from build123d import *

# Parameters (mm, degrees)
SKETCH_1_W           = 44
SKETCH_1_H           = 81
EXTRUDE_1_DEPTH      = 25
SHELL_1_T            = -2
FILLET_1_R           = 2
SKETCH_2_R           = 0.8
SKETCH_2_R_2         = 0.9
CUT_EXTRUDE_1_DEPTH  = 24
SKETCH_3_R           = 1.25
CUT_EXTRUDE_2_DEPTH  = 24
SKETCH_4_R           = 6
EXTRUDE_2_DEPTH      = 2
CUT_EXTRUDE_START    = -13.2
SKETCH_6_R           = 1.25
CUT_EXTRUDE_4_DEPTH  = 13.2
SKETCH_7_W           = 15.5
SKETCH_7_H           = 17.5
CUT_EXTRUDE_5_DEPTH  = 13.2
SKETCH_9_W           = 18.8
SKETCH_9_H           = 6.5
SKETCH_9_R           = 0.9
EXTRUDE_3_DEPTH      = 8
SKETCH_11_W          = 11
SKETCH_11_H          = 6.5
CUT_EXTRUDE_6_DEPTH  = 4
SKETCH_12_W          = 10
SKETCH_12_H          = 3.5
CUT_EXTRUDE_7_DEPTH  = 4
FILLET_2_R           = 2
EXTRUDE_START        = -1
SKETCH_14_R          = 1.25
EXTRUDE_4_DEPTH      = 1
SKETCH_15_R          = 2
CUT_EXTRUDE_8_DEPTH  = 1
SKETCH_17_R          = 2
EXTRUDE_5_DEPTH      = 3
SKETCH_18_R          = 0.85
CUT_EXTRUDE_10_DEPTH = 3
FILLET_4_R           = 1


with BuildPart() as part:
    # 草图1 → 凸台-拉伸1 (new body)
    with BuildSketch(Plane(origin=(0, 0, 0), x_dir=(1, 0, 0), z_dir=(0, 1, 0))):
        with Locations((0, -2.5)):
            Rectangle(SKETCH_1_W, SKETCH_1_H)
    extrude(amount=EXTRUDE_1_DEPTH)

    # 抽壳1
    shell_1_openings = [part.faces().sort_by_distance(p)[0] for p in [
        (0, 25, 2.5),
    ]]
    offset(amount=SHELL_1_T, openings=shell_1_openings, kind=Kind.INTERSECTION)

    # 圆角1
    fillet_1_edges = [part.edges().sort_by_distance(p)[0] for p in [
        (0, 0, -38),
        (22, 0, 2.5),
        (0, 0, 43),
        (-22, 0, 2.5),
        (-22, 12.5, -38),
        (22, 12.5, -38),
        (22, 12.5, 43),
        (-22, 12.5, 43),
    ]]
    fillet(fillet_1_edges, radius=FILLET_1_R)

    # 草图2 → 切除-拉伸1 (cut)
    with BuildSketch(Plane(origin=(0, 2, 0), x_dir=(1, 0, 0), z_dir=(0, 1, 0))):
        with Locations(Location((4.8, 16.9, 0), (0, 0, 270))):
            Circle(SKETCH_2_R)
        with Locations(Location((16.1, -9.5, 0), (0, 0, 270))):
            Circle(SKETCH_2_R_2)
    extrude(amount=-CUT_EXTRUDE_1_DEPTH, mode=Mode.SUBTRACT)

    # 草图3 → 切除-拉伸2 (cut)
    with BuildSketch(Plane(origin=(0, 2, 0), x_dir=(1, 0, 0), z_dir=(0, 1, 0))):
        with Locations(Location((-9.5, -3, 0), (0, 0, 270))):
            Circle(SKETCH_3_R)
    extrude(amount=-CUT_EXTRUDE_2_DEPTH, mode=Mode.SUBTRACT)

    # 草图4 → 凸台-拉伸2 (add)
    with BuildSketch(Plane(origin=(0, 2, 0), x_dir=(1, 0, 0), z_dir=(0, 1, 0))):
        with Locations(Location((-9.5, -3, 0), (0, 0, 270))):
            Circle(SKETCH_4_R)
    extrude(amount=EXTRUDE_2_DEPTH)

    # 草图6 → 切除-拉伸4 (cut)
    with BuildSketch(Plane.XZ.offset(CUT_EXTRUDE_START)):
        with Locations(Location((-9.5, 3, 0), (0, 0, 90))):
            Circle(SKETCH_6_R)
    extrude(amount=CUT_EXTRUDE_4_DEPTH, mode=Mode.SUBTRACT)

    # 草图7 → 切除-拉伸5 (cut)
    with BuildSketch(Plane(origin=(0, 0, -38), x_dir=(-1, 0, 0), z_dir=(0, 0, -1))):
        with Locations((-10.25, 12.5)):
            Rectangle(SKETCH_7_W, SKETCH_7_H)
    extrude(amount=-CUT_EXTRUDE_5_DEPTH, mode=Mode.SUBTRACT)

    # 草图9 → 凸台-拉伸3 (add)
    with BuildSketch(Plane(origin=(0, 2, 0), x_dir=(1, 0, 0), z_dir=(0, 1, 0))):
        with Locations((10.6, -37.75)):
            Rectangle(SKETCH_9_W, SKETCH_9_H)
        with Locations(Location((18.1, -37.9, 0), (0, 0, 270))):
            Circle(SKETCH_9_R, mode=Mode.SUBTRACT)
        with Locations(Location((3.1, -37.9, 0), (0, 0, 270))):
            Circle(SKETCH_9_R, mode=Mode.SUBTRACT)
    extrude(amount=EXTRUDE_3_DEPTH)

    # 草图11 → 切除-拉伸6 (cut)
    with BuildSketch(Plane(origin=(0, 10, 0), x_dir=(1, 0, 0), z_dir=(0, 1, 0))):
        with Locations((10.6, -37.75)):
            Rectangle(SKETCH_11_W, SKETCH_11_H)
    extrude(amount=-CUT_EXTRUDE_6_DEPTH, mode=Mode.SUBTRACT)

    # 草图12 → 切除-拉伸7 (cut)
    with BuildSketch(Plane.XY.offset(43)):
        with Locations((10.6, 10)):
            Rectangle(SKETCH_12_W, SKETCH_12_H)
    extrude(amount=-CUT_EXTRUDE_7_DEPTH, mode=Mode.SUBTRACT)

    # 圆角2
    fillet_2_edges = [part.edges().sort_by_distance(p)[0] for p in [
        (10.6, 2, 34.5),
        (1.2, 2, 37.75),
        (1.2, 6, 34.5),
    ]]
    fillet(fillet_2_edges, radius=FILLET_2_R)

    # 草图14 → 凸台-拉伸4 (add)
    with BuildSketch(Plane.XZ.offset(EXTRUDE_START)):
        with Locations(Location((-9.5, 3, 0), (0, 0, 90))):
            Circle(SKETCH_14_R)
    extrude(amount=EXTRUDE_4_DEPTH)

    # 草图15 → 切除-拉伸8 (cut)
    with BuildSketch(Plane.XZ):
        with Locations(Location((16.1, 9.5, 0), (0, 0, 270))):
            Circle(SKETCH_15_R)
        with Locations(Location((4.8, -16.9, 0), (0, 0, 270))):
            Circle(SKETCH_15_R)
    extrude(amount=-CUT_EXTRUDE_8_DEPTH, mode=Mode.SUBTRACT)

    # 草图17 → 凸台-拉伸5 (add)
    with BuildSketch(Plane(origin=(0, 25, 0), x_dir=(1, 0, 0), z_dir=(0, 1, 0))):
        with Locations((19, 35)):
            Circle(SKETCH_17_R)
        with Locations((-19, 35)):
            Circle(SKETCH_17_R)
        with Locations((-19, -40)):
            Circle(SKETCH_17_R)
        with Locations((19, -40)):
            Circle(SKETCH_17_R)
    extrude(amount=-EXTRUDE_5_DEPTH)

    # 草图18 → 切除-拉伸10 (cut)
    with BuildSketch(Plane(origin=(0, 25, 0), x_dir=(1, 0, 0), z_dir=(0, 1, 0))):
        with Locations(Location((19, 35, 0), (0, 0, 270))):
            Circle(SKETCH_18_R)
        with Locations(Location((-19, 35, 0), (0, 0, 90))):
            Circle(SKETCH_18_R)
        with Locations(Location((-19, -40, 0), (0, 0, 270))):
            Circle(SKETCH_18_R)
        with Locations(Location((19, -40, 0), (0, 0, 90))):
            Circle(SKETCH_18_R)
    extrude(amount=-CUT_EXTRUDE_10_DEPTH, mode=Mode.SUBTRACT)

    # 圆角4
    fillet_4_edges = [part.edges().sort_by_distance(p)[0] for p in [
        (17.267949192, 23.5, -36),
        (20, 23.5, -33.267949192),
        (-17.267949192, 23.5, -36),
        (-20, 23.5, -33.267949192),
        (-20, 23.5, 38.267949192),
        (-17.267949192, 23.5, 41),
        (17.267949192, 23.5, 41),
        (20, 23.5, 38.267949192),
    ]]
    fillet(fillet_4_edges, radius=FILLET_4_R)


solid = part.part
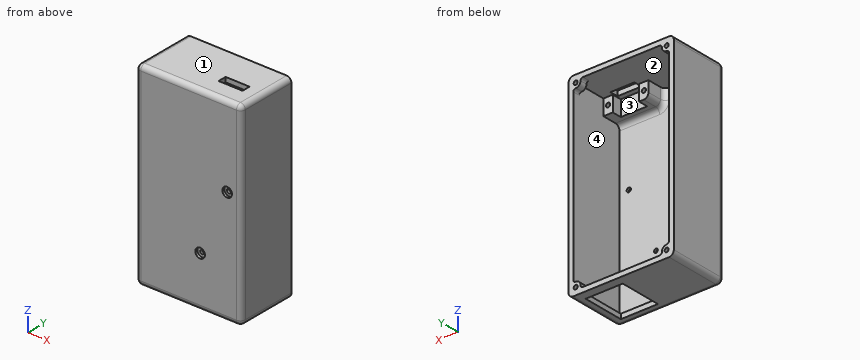
Geometry: final body of the model. Coordinates: model frame, mm. Face numbers are marked on the shaded views. Give positions to 0.01 mm unless a question says otherwise; leave off trailing zeros. Write each loop counter-clockwise with the first axis right and the second up, starting at its lowest first coordinate (ties: lowest second). Pieces come first, ordered by that corner, then holes. Notation, with made-up numbers: (82.25, 83) -> (94.25, 83) arc R20 cw to (94.25, 94) -> close; hole circle Ø2 at (-33, 50.25). An arc over 180 degrees is marked (long way). Answer as a JSON object with one key per item and string values.
1. Mould query, pull axis Z, two halves, no side actions, for the marked faces 1, 2, 3 and 4. Classes: pulls with the +Z half, pulls with the -Z half, needs draft (parallel to the pull), parting line crosses it, or undercut.
Ans:
{"face 1": "pulls with the +Z half", "face 2": "undercut", "face 3": "needs draft", "face 4": "undercut"}
2. Cut plane C-C on y = 15. Output: boundary loops of the cut face in (x, z).
Ans:
{"outline": "(-22, -36) arc R2 ccw to (-20, -38) -> (2.5, -38) -> (2.5, -36) -> (-20, -36) -> (-20, 41) -> (20, 41) -> (20, -36) -> (18, -36) -> (18, -38) -> (20, -38) arc R2 ccw to (22, -36) -> (22, 41) arc R2 ccw to (20, 43) -> (-20, 43) arc R2 ccw to (-22, 41) -> close"}
3. Cut plane B-B on z = -16.9. Output: boundary loops of the cut face in (x, y), and give its area (3 significant figures).
Ans:
{"outline": "(-22, 2) arc R2 ccw to (-20, 0) -> (2.8, 0) -> (2.8, 1) -> (4, 1) -> (4, 2) -> (-20, 2) -> (-20, 25) -> (-22, 25) -> close; (5.6, 1) -> (6.8, 1) -> (6.8, 0) -> (20, 0) arc R2 ccw to (22, 2) -> (22, 25) -> (20, 25) -> (20, 2) -> (5.6, 2) -> close", "area": "173 mm^2"}
4. Cut plane A-A on x = 9.5. Output: boundary loops of the cut face in (y, z).
Ans:
{"outline": "(0, -36) arc R2 ccw to (2, -38) -> (3.75, -38) -> (3.75, -36) -> (2, -36) -> (2, 32.5) arc R2 cw to (4, 34.5) -> (6, 34.5) -> (6, 41) -> (8.25, 41) -> (8.25, 43) -> (2, 43) arc R2 ccw to (0, 41) -> close; (11.75, 41) -> (25, 41) -> (25, 43) -> (11.75, 43) -> close; (21.25, -38) -> (25, -38) -> (25, -36) -> (21.25, -36) -> close"}
5. Cut plane D-D on x = -9.5. Output: boundary loops of the cut face in (y, z).
Ans:
{"outline": "(0, -36) arc R2 ccw to (2, -38) -> (25, -38) -> (25, -36) -> (2, -36) -> (2, -3) -> (4, -3) -> (4, 1.75) -> (1, 1.75) -> (1, 4.25) -> (4, 4.25) -> (4, 9) -> (2, 9) -> (2, 41) -> (25, 41) -> (25, 43) -> (2, 43) arc R2 ccw to (0, 41) -> close"}
6. Contact query for flat-ended pins moving along their axis: pin 1 (3 mm diameter, centred on x = -3.5, z = 22, fed in from +Y); pin 2 (0.8 mm diameter, centred on x = -9.5, z = 3.5, fed in from +Y); pin 3 (2.5 mm diameter, centred on x = 3.1, z = 37.9, fed in from +Y). Output: stop coordinate, or through.
Ans:
{"pin 1": "stops at y = 2", "pin 2": "stops at y = 1", "pin 3": "stops at y = 10"}
7. Ray query, probe 1 along X at (y, z) = (24.4, 40); probe 2 along X at (y, z) = (9.5, -12); probe 3 along X at (y, z) = (6.5, 37.9). Return the intervals inside material, ascending. Write a range as from..to.
Ans:
{"probe 1": "x = -22..-19.85, -18.15..-17, 17..18.15, 19.85..22", "probe 2": "x = -22..-20, 20..22", "probe 3": "x = -22..-20, 1.2..2.2, 4..5.1, 16.1..17.2, 19..22"}
